Geometry check sheet. Reference: the model listing, model coordinates, mm. A direction names the side the tool comes from. Give positions to 0.01 mm unless a question says otherwise; leave off trailing zeros. Write each loop counter-clockwise with the first axis right and the second up, starting at its lowest first coordinate (ties: lowest second). Pieces come first, ordered by that corner, then holes.
(1) Cross-section at B-B (x = -38.1). Record the boundary of the cut face in (y, z).
(2) Depth check by flat-ended pin: P1, Ø3, axis at x = -5.5, z = 1.5, coming from the +Y side; P2, Ø1.5, axis at x = -56, z = 3, coming from the +Y side; P3, Ø6.5, axis at x = -12.7, y = 152.4, coming from the -Z side. Enter the tip coordinate at first touch or a pass-through.
(3) Thickness scan on line 1 along X through (y, z) = (152.4, 2) (3 decimals); line 2 along X through (y, z) = (138, 5.5) (3 decimals). Record the ranges inside material, lowest first.
(4) Cross-section at A-A (y = 152.4). Record the boundary of the cut face in (x, z) (3 decimals).
(5) Cross-section at C-C (z = 4.25). Count the separate pieces of the cut face and the enclosed holes in it, and give its area (3 significant figures).
(6) Mould release check, pull along X, two halves, no side actions. Record for faces 4 (the flat face through (-146.05, 130, 3)), 5 (the cylindrical face through (82.619, 282.555, 3.131)), 6 (the flat face through (-35, 149, 0)), 7 (the cylindrical face through (-12.24, 47.26, 3.13)): +X half, -X half, draft (parallel to the pull), parting line (faces both ways), or undercut.
(7) Cross-section at D-D (x = 124). Record the boundary of the cut face in (y, z).
(8) Tool access check on faces 1 (the flat face through (3.175, 110, 3)), 2 (the cylindrical face through (36.18, 47.79, 3.13)), 3 (the flat face through (0, 281.412, 3)). Record the directions out of +Z, -Z, +X, -X, +Y, -Y that give a thin tool (end or side, any length) a straight path to the whole face; none if there is none.
```python
from build123d import *

# Parameters (mm, degrees)
BOSS_EXTRUDE2_DEPTH     = 6.35
CUT_EXTRUDE3_DEPTH      = 148.336
CUT_EXTRUDE3_DEPTH_BACK = 93.472
SKETCH3_R               = 3.5687


with BuildPart() as part:
    # Sketch2 → Boss-Extrude2 (new body)
    with BuildSketch(Plane.XY):
        with BuildLine():
            Line((-3.175, 0), (-3.175, 217.911929367))
            Line((-3.175, 217.911929367), (3.175, 217.911929367))
            Line((3.175, 217.911929367), (3.175, 0))
            Line((3.175, 0), (146.05, 0))
            Line((146.05, 0), (146.05, 255.602258394))
            ThreePointArc((146.05, 255.602258394), (81.677042764, 282.828530529), (12.7, 294.111929367))
            Line((12.7, 294.111929367), (12.7, 281.411929367))
            Line((12.7, 281.411929367), (-12.7, 281.411929367))
            Line((-12.7, 281.411929367), (-12.7, 294.111929367))
            ThreePointArc((-12.7, 294.111929367), (-81.677042764, 282.828530529), (-146.05, 255.602258394))
            Line((-146.05, 255.602258394), (-146.05, 0))
            Line((-146.05, 0), (-3.175, 0))
        make_face()
    extrude(amount=BOSS_EXTRUDE2_DEPTH)

    # Sketch3 → Cut-Extrude3 (cut, two sides: drawn at the far end of the back side and taken through both)
    with BuildSketch(Plane.XY.offset(-CUT_EXTRUDE3_DEPTH_BACK)):
        with Locations(Location((12.7, 50.8, 0), (0, 0, 180))):
            Circle(SKETCH3_R)
        with Locations(Location((38.1, 50.8, 0), (0, 0, 180))):
            Circle(SKETCH3_R)
        with Locations(Location((12.7, 152.4, 0), (0, 0, 180))):
            Circle(SKETCH3_R)
        with Locations(Location((38.1, 152.4, 0), (0, 0, 180))):
            Circle(SKETCH3_R)
        with Locations(Location((-12.7, 50.8, 0), (0, 0, 180))):
            Circle(SKETCH3_R)
        with Locations(Location((-38.1, 50.8, 0), (0, 0, 180))):
            Circle(SKETCH3_R)
        with Locations(Location((-38.1, 152.4, 0), (0, 0, 180))):
            Circle(SKETCH3_R)
        with Locations(Location((-12.7, 152.4, 0), (0, 0, 180))):
            Circle(SKETCH3_R)
    extrude(amount=CUT_EXTRUDE3_DEPTH + CUT_EXTRUDE3_DEPTH_BACK, mode=Mode.SUBTRACT)


solid = part.part
```
Reply:
1. outline: (0, 0) - (47.23, 0) - (47.23, 6.35) - (0, 6.35) - close; (54.37, 0) - (148.83, 0) - (148.83, 6.35) - (54.37, 6.35) - close; (155.97, 0) - (291.91, 0) - (291.91, 6.35) - (155.97, 6.35) - close
2. P1: stops at y = 281.41
2. P2: stops at y = 289.15
2. P3: passes through
3. line 1: x = -146.05 to -41.669, -34.531 to -16.269, -9.131 to -3.175, 3.175 to 9.131, 16.269 to 34.531, 41.669 to 146.05
3. line 2: x = -146.05 to -3.175, 3.175 to 146.05
4. outline: (-146.05, 0) - (-41.669, 0) - (-41.669, 6.35) - (-146.05, 6.35) - close; (-34.531, 0) - (-16.269, 0) - (-16.269, 6.35) - (-34.531, 6.35) - close; (-9.131, 0) - (-3.175, 0) - (-3.175, 6.35) - (-9.131, 6.35) - close; (3.175, 0) - (9.131, 0) - (9.131, 6.35) - (3.175, 6.35) - close; (16.269, 0) - (34.531, 0) - (34.531, 6.35) - (16.269, 6.35) - close; (41.669, 0) - (146.05, 0) - (146.05, 6.35) - (41.669, 6.35) - close
5. separate pieces: 1
5. enclosed holes: 8
5. area: 80,300 mm2
6. face 4: -X half
6. face 5: +X half
6. face 6: draft
6. face 7: undercut
7. outline: (0, 0) - (267, 0) - (267, 6.35) - (0, 6.35) - close
8. face 1: +Z, -Z, -Y
8. face 2: +Z, -Z
8. face 3: +Z, -Z, +Y
